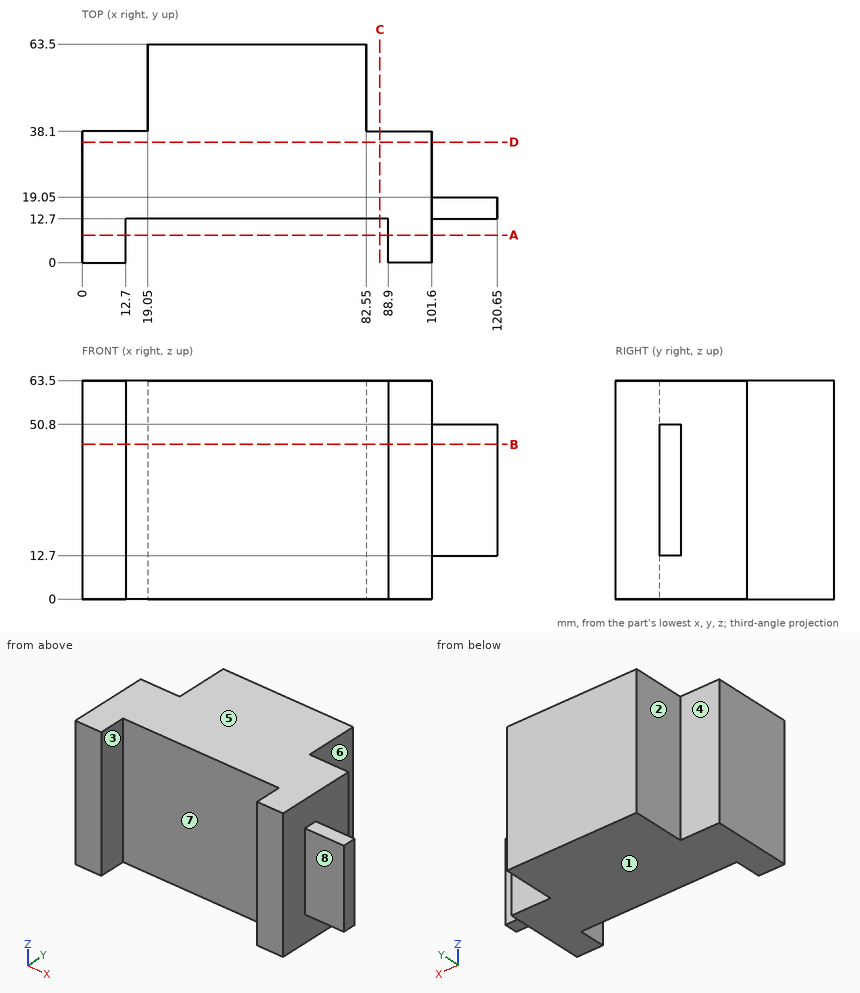
Geometry: see drawing. Coordinates: mm, zero at the bounding-box minimum. A direction names the side the tool comes from. Coordinates: 2 decimals unless noted, no trailing zeros. Write each loop counter-clockwise with the first axis right and the second up, starting at its lowest first coordinate (ties: lowest second). Pieces come first, ordered by that corner, then holes. Notation, with made-up numbers: M 51,7 L 76,7 A9 cw 76,11 Z; hole C -20,24 d7. An arc over 180 degrees is marked long. Use CSV: the item, a comma, the result in double quotes. Start each with the question number.
1. Cut plane B-B on z = 45. Return the cut outline in (x, y).
2. Mould query, pull axis X, two halves, no side actions, for the marked faces 1, 2 and 3. Classes: pulls with the +X half, pulls with the -X half, needs draft (parallel to the pull), parting line crosses it, or undercut.
3. Cut plane D-D on y = 35. Return the cut outline in (x, z), plus the area to 3 significant figures.
4. Ray query, probe 1 along X at (y, z) = (11, 4.5); probe 2 along Y at (x, z) = (36, 9); probe 3 along X at (y, z) = (53, 29.5). Return the intervals inside material, ascending.
5. Reachability of the marked faces 4, 5, 6, 7 and 8 from +Z, -Z, +X, -X, +Y, -Y: full face, straight path, thin tool, end or side. Return the list, or none.
6. First-contact query: P1, Ø1.5, axis at x = 60, z = 38.5, coming from the -Y side; P2, Ø8, axis at x = 94, z = 19, coming from the +Y side; P3, Ø1.9, axis at x = 110.5, y = 17.5, coming from the +Z side. Flat tips, straight axial feed; report the tip coordinate or a pass-through.
7. Cut plane A-A on y = 8. Return the cut outline in (x, z), plus the area to 3 significant figures.
8. Cut plane C-C on x = 86.5. Return the cut outline in (y, z), plus the area to 3 significant figures.
Entries:
1,outline,"M 0,0 L 12.7,0 L 12.7,12.7 L 88.9,12.7 L 88.9,0 L 101.6,0 L 101.6,12.7 L 120.65,12.7 L 120.65,19.05 L 101.6,19.05 L 101.6,38.1 L 82.55,38.1 L 82.55,63.5 L 19.05,63.5 L 19.05,38.1 L 0,38.1 Z"
2,face 1,"needs draft"
2,face 2,"pulls with the -X half"
2,face 3,"undercut"
3,outline,"M 0,0 L 101.6,0 L 101.6,63.5 L 0,63.5 Z"
3,area,"6,450 mm²"
4,probe 1,"0 to 12.7, 88.9 to 101.6"
4,probe 2,"12.7 to 63.5"
4,probe 3,"19.05 to 82.55"
5,face 4,"+Z, -Z, -X, +Y"
5,face 5,"+Z, +X, -X, +Y, -Y"
5,face 6,"+Z, -Z, +X, +Y"
5,face 7,"+Z, -Z, -Y"
5,face 8,"+Z, -Z, +X, -Y"
6,P1,"y = 12.7"
6,P2,"y = 38.1"
6,P3,"z = 50.8"
7,outline,"M 0,0 L 12.7,0 L 12.7,63.5 L 0,63.5 Z; M 88.9,0 L 101.6,0 L 101.6,63.5 L 88.9,63.5 Z"
7,area,"1,610 mm²"
8,outline,"M 12.7,0 L 38.1,0 L 38.1,63.5 L 12.7,63.5 Z"
8,area,"1,610 mm²"
